Geometry check sheet. Reference: the model listing, model coordinates, mm. Face numbers are marked on the shaded views. A direction names the side the tool comes from. Round coordinates to 2 decimals unless told otherwise and drop trailing zeros. Loops run counter-clockwise (first coordinate to the right, second up) from the corner with the lowest first, then second, coordinate; pieces in that order, holes last.
```python
from build123d import *

# Parameters (mm, degrees)
SKETCH1_W           = 250
SKETCH1_H           = 220
SKETCH1_W_2         = 244
SKETCH1_H_2         = 214
EXTRUDE_THIN1_DEPTH = 40
FILLET1_R           = 3


with BuildPart() as part:
    # Sketch1 → Extrude-Thin1 (new body)
    with BuildSketch(Plane.XY):
        with Locations((35.461157826, 79.854863969)):
            Rectangle(SKETCH1_W, SKETCH1_H)
        with Locations((35.461157826, 79.854863969)):
            Rectangle(SKETCH1_W_2, SKETCH1_H_2, mode=Mode.SUBTRACT)
    extrude(amount=EXTRUDE_THIN1_DEPTH)

    # Fillet1
    fillet1_edges = [part.edges().sort_by_distance(p)[0] for p in [
        (160.461157826, -30.145136031, 20),
        (-89.538842174, -30.145136031, 20),
        (-89.538842174, 189.854863969, 20),
        (160.461157826, 189.854863969, 20),
    ]]
    fillet(fillet1_edges, radius=FILLET1_R)


solid = part.part
```
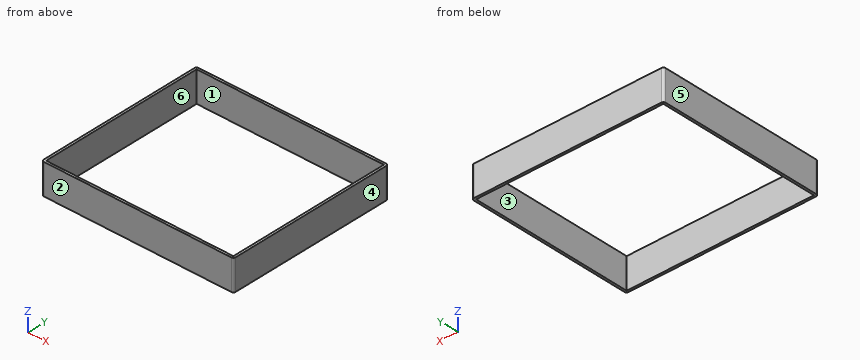
1) Mould release check, pull along X, two halves, no side actions. Record for the marked faces 3, 4, 5 and 6: +X half, -X half, draft (parallel to the pull), parting line (faces both ways), or undercut.
Report:
face 3: undercut
face 4: +X half
face 5: -X half
face 6: undercut
2) Sectioned sample at A-A, the plane x = 8.5. Record the cut outline in (y, z), then the cut area to 3 significant figures.
Report:
outline: (-30.15, 0) - (-27.15, 0) - (-27.15, 40) - (-30.15, 40) - close; (186.85, 0) - (189.85, 0) - (189.85, 40) - (186.85, 40) - close
area: 240 mm2
3) Sectioned sample at C-C, the plane z = 22. Record the cut outline in (x, y), then the cut area to 3 significant figures.
Report:
outline: (-89.54, -27.15) arc R3 ccw to (-86.54, -30.15) - (157.46, -30.15) arc R3 ccw to (160.46, -27.15) - (160.46, 186.85) arc R3 ccw to (157.46, 189.85) - (-86.54, 189.85) arc R3 ccw to (-89.54, 186.85) - close; hole (-86.54, -27.15) - (157.46, -27.15) - (157.46, 186.85) - (-86.54, 186.85) - close
area: 2,780 mm2
4) Sectioned sample at B-B, the plane y = 122. Record the cut outline in (x, z).
Report:
outline: (-89.54, 0) - (-86.54, 0) - (-86.54, 40) - (-89.54, 40) - close; (157.46, 0) - (160.46, 0) - (160.46, 40) - (157.46, 40) - close
5) Access from +Z, -Z, +X, -X, +Y, -Y to the whole of each face (thin tool, end or side, straight path). Record for the marked faces 1 and 2.
Report:
face 1: +Z, -Z
face 2: +Z, -Z, +X, -X, -Y
6) Scan lines: line 1 along X through (y, z) = (28.5, 25.5); line 2 along Y through (x, z) = (114, 17). Record each from-to range of solid material in increasing order.
Report:
line 1: x = -89.54 to -86.54, 157.46 to 160.46
line 2: y = -30.15 to -27.15, 186.85 to 189.85
